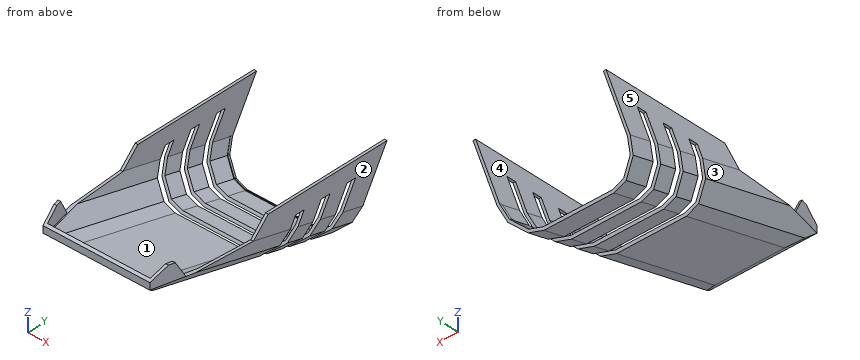
```python
from build123d import *
from OCP.BRepFilletAPI import BRepFilletAPI_MakeChamfer

# Parameters (mm, degrees)
BOSS_EXTRU_1_DEPTH                  = 500
CHANFREIN2_SIZE                     = 80
CHANFREIN3_SIZE                     = 19.999999999999996
CHANFREIN3_SIZE2                    = 38.63703305156302
CHANFREIN3_SIZE2_2                  = 38.63703305156301
CHANFREIN4_SIZE                     = 190.00000000000003
CHANFREIN4_SIZE2                    = 127.87558157978762
BOSS_EXTRU_2_DEPTH                  = 60
BOSS_EXTRU_3_DEPTH                  = 500
COQUE1_T                            = 10
ENL_V_MAT_EXTRU_2_REACH             = 940.137
ENL_V_MAT_EXTRU_2_DIRECTION_2_DEPTH = 939.1366191668232
ENL_V_START                         = -60
ENL_V_MAT_EXTRU_3_DEPTH             = 60
ENL_V_MAT_EXTRU_4_DEPTH             = 1170.3404261816813
CHANFREIN6_SIZE                     = 34.641016151
CHANFREIN6_SIZE_2                   = 60
CHANFREIN7_SIZE                     = 60
ENL_V_MAT_EXTRU_5_DEPTH             = 1170.3404261816813


# Some blends are built 0.0001 mm under size
with BuildPart() as part:
    # Esquisse3 → Boss.-Extru.1 (new body)
    with BuildSketch(Plane(origin=(0, 0, 0), x_dir=(0, 0, -1), z_dir=(1, 0, 0))):
        Polygon((0, 0), (0, 1000), (216.50635094611002, 875.0000000000006), align=None)
    extrude(amount=BOSS_EXTRU_1_DEPTH)

    # Chanfrein2
    chanfrein2_edges = [part.edges().sort_by_distance(p)[0] for p in [
        (500, 437.5000000000003, -108.25317547305501),
        (0, 437.5000000000003, -108.25317547305501),
    ]]
    chamfer(chanfrein2_edges, length=CHANFREIN2_SIZE)

    # Chanfrein3: one chamfer whose edges measure the first distance from different faces: ONE call of the kernel's chamfer builder (chamfer() names one face for all edges)
    chanfrein3_edges_1 = [part.edges().sort_by_distance(p)[0] for p in [
        (500, 624.8499399519503, -72.19766271841472),
        (420, 437.5000000000003, -108.25317547305504),
    ]]
    chanfrein3_side_1 = [part.faces().sort_by_distance(p)[0] for p in [
        (457.3358939482921, 524.9359686158087, -91.42611546732361),
    ]]
    chanfrein3_edges_2 = [part.edges().sort_by_distance(p)[0] for p in [
        (80, 437.50000000000017, -108.25317547305501),
        (0, 624.8499399519503, -72.1976627184147),
    ]]
    chanfrein3_side_2 = [part.faces().sort_by_distance(p)[0] for p in [
        (42.664106051707925, 524.9359686158089, -91.42611546732363),
    ]]
    chanfrein3 = BRepFilletAPI_MakeChamfer(part.part.solid().wrapped)
    for e in chanfrein3_edges_1:
        chanfrein3.Add(CHANFREIN3_SIZE, CHANFREIN3_SIZE2, e.wrapped, chanfrein3_side_1[0].wrapped)  # the first distance lies on this face
    for e in chanfrein3_edges_2:
        chanfrein3.Add(CHANFREIN3_SIZE, CHANFREIN3_SIZE2_2, e.wrapped, chanfrein3_side_2[0].wrapped)  # the first distance lies on this face
    add(Compound.cast(chanfrein3.Shape()), mode=Mode.REPLACE)

    # Chanfrein4
    chanfrein4_edges = [part.edges().sort_by_distance(p)[0] for p in [
        (249.99999999999994, 0, 0),
    ]]
    chanfrein4_side = [part.faces().sort_by_distance(p)[0] for p in [
        (249.99999999999997, 437.5000000000003, -108.25317547305502),
    ]]
    chamfer(chanfrein4_edges, length=CHANFREIN4_SIZE, length2=CHANFREIN4_SIZE2, reference=chanfrein4_side[0])

    # Esquisse4 → Boss.-Extru.2 (add)
    with BuildSketch(Plane.XY):
        Polygon((500, 1000), (0, 1000), (6.94e-15, 493.9253559619593), (14.142135623731011, 274.1881541390633), (49.28527880731526, 127.87558157978796), (450.7147211926849, 127.87558157978796), (485.85786437626905, 274.18815413906196), (500, 493.92535596195466), align=None)
    extrude(amount=BOSS_EXTRU_2_DEPTH)

    # Esquisse5 → Boss.-Extru.3 (add)
    with BuildSketch(Plane.ZY):
        Polygon((60, 1000), (60, 1034.6410161513777), (0, 1000), align=None)
    extrude(amount=-BOSS_EXTRU_3_DEPTH)

    # Coque1 (no face opened: a closed hollow body)
    add(offset(amount=-COQUE1_T, mode=Mode.PRIVATE), mode=Mode.SUBTRACT)

    # Esquisse6 → Enlèv. mat.-Extru.2 (cut, up to next)
    with BuildSketch(Plane(origin=(0, 750.0000000000025, -433.0127018922181), x_dir=(1, 0, 0), z_dir=(0, 0.86602540378444, -0.49999999999999784)), mode=Mode.PRIVATE) as enl_v_mat_extru_2_sk1:
        Polygon((10, -569.2820323027529), (10, -757.501187283232), (489.99999999999983, -757.5011872832318), (489.99999999999994, -569.2820323027527), (489.9999999999996, -374.7478772728107), (476.8280711810083, -323.58228852611177), (428.823967356419, -273.61803314286686), (379.9946243192759, -259.99999999999744), (120.00537568072383, -259.99999999999756), (71.17603264358065, -273.618033142867), (23.171928818991503, -323.58228852611194), (10.000000000000268, -374.74787727281085), align=None)
    enl_v_mat_extru_2_tool1 = extrude(enl_v_mat_extru_2_sk1.sketch, amount=-ENL_V_MAT_EXTRU_2_REACH, mode=Mode.PRIVATE) & part.part
    add(enl_v_mat_extru_2_tool1.solids().sort_by_distance((250, 1007.562635, 13.098868))[0], mode=Mode.SUBTRACT)

    # Esquisse6 → Enlèv. mat.-Extru.2 direction 2 (cut)
    with BuildSketch(Plane(origin=(0, 750.0000000000025, -433.0127018922181), x_dir=(1, 0, 0), z_dir=(0, 0.86602540378444, -0.49999999999999784))):
        Polygon((10, -569.2820323027529), (10, -757.501187283232), (489.99999999999983, -757.5011872832318), (489.99999999999994, -569.2820323027527), (489.9999999999996, -374.7478772728107), (476.8280711810083, -323.58228852611177), (428.823967356419, -273.61803314286686), (379.9946243192759, -259.99999999999744), (120.00537568072383, -259.99999999999756), (71.17603264358065, -273.618033142867), (23.171928818991503, -323.58228852611194), (10.000000000000268, -374.74787727281085), align=None)
    extrude(amount=ENL_V_MAT_EXTRU_2_DIRECTION_2_DEPTH, mode=Mode.SUBTRACT)

    # Esquisse7 → Enlèv. mat.-Extru.3 (cut)
    with BuildSketch(Plane.XY.offset(60).offset(ENL_V_START)):
        Polygon((475.93370620438793, 275.68803078848794), (442.8322266096682, 137.87558157978802), (57.16777339033198, 137.87558157978796), (24.066293795611983, 275.6880307884899), (10.000000000000009, 494.2468199914388), (10, 1034.6410161513777), (489.99999999999864, 1034.6410161513782), (489.9999999999996, 494.2468199914393), align=None)
    extrude(amount=ENL_V_MAT_EXTRU_3_DEPTH, mode=Mode.SUBTRACT)

    # Esquisse8 → Enlèv. mat.-Extru.4 (cut, through all)
    with BuildSketch(Plane(origin=(500, 0, 0), x_dir=(0, 0, -1), z_dir=(1, 0, 0))):
        Polygon((-60, 493.92535596195466), (0, 493.92535596195466), (-1.388e-14, 274.18815413906196), (-1.388e-14, 244.18815413906194), (-59.99999999999999, 244.18815413906194), (-60, 274.18815413906196), align=None)
    extrude(amount=-ENL_V_MAT_EXTRU_4_DEPTH, mode=Mode.SUBTRACT)

    # Chanfrein6
    # the kernel refuses this chamfer: 60, 34.641016151 mm, written as the material it takes off along each edge
    with BuildSketch(Plane(origin=(186.85746471381282, 244.1881541390619, 60), x_dir=(0, -0.9983227437537926, 0.05789386240267061), z_dir=(-1, 0, 0))) as chanfrein6_piece_1_section:
        Polygon((CHANFREIN6_SIZE * 0.998322743765, -CHANFREIN6_SIZE * 0.0578938624033), (-CHANFREIN6_SIZE_2 * 0.0578938624027, -CHANFREIN6_SIZE_2 * 0.998322743754), (0, 0), align=None)
    chanfrein6_piece_1 = extrude(amount=320.73470744761204, mode=Mode.PRIVATE)
    chanfrein6_piece_1 = split(chanfrein6_piece_1, bisect_by=Plane(origin=(26.49011099000677, 233.04123739645672, 1.648e-14), z_dir=(0, 6e-17, 1)), keep=Keep.TOP, mode=Mode.PRIVATE)
    add(chanfrein6_piece_1, mode=Mode.SUBTRACT)
    with BuildSketch(Plane(origin=(-105.93986647144428, 127.87558157978796, 60), x_dir=(0, -0.05789386240267084, -0.9983227437537926), z_dir=(1, 0, 0))) as chanfrein6_piece_2:
        Polygon((CHANFREIN6_SIZE * 0.998322743765, CHANFREIN6_SIZE * 0.0578938624033), (-CHANFREIN6_SIZE_2 * 0.0578938624027, CHANFREIN6_SIZE_2 * 0.998322743754), (0, 0), align=None)
    extrude(amount=711.8797329428887, mode=Mode.SUBTRACT)
    with BuildSketch(Plane(origin=(633.8772427337997, 244.1881541390619, 60), x_dir=(0, -0.9983227437537926, 0.05789386240267061), z_dir=(-1, 0, 0))) as chanfrein6_piece_3_section:
        Polygon((CHANFREIN6_SIZE * 0.998322743765, -CHANFREIN6_SIZE * 0.0578938624033), (-CHANFREIN6_SIZE_2 * 0.0578938624027, -CHANFREIN6_SIZE_2 * 0.998322743754), (0, 0), align=None)
    chanfrein6_piece_3 = extrude(amount=320.7347074476121, mode=Mode.PRIVATE)
    chanfrein6_piece_3 = split(chanfrein6_piece_3, bisect_by=Plane(origin=(473.5098890099937, 233.04123739645678, 1.648e-14), z_dir=(0, 6e-17, 1)), keep=Keep.TOP, mode=Mode.PRIVATE)
    add(chanfrein6_piece_3, mode=Mode.SUBTRACT)

    # Chanfrein7
    chanfrein7_edges = [part.edges().sort_by_distance(p)[0] for p in [
        (5.010344602246278, 493.92535596195466, 60),
        (494.98965539775355, 493.92535596195466, 60),
    ]]
    chamfer(chanfrein7_edges, length=CHANFREIN7_SIZE - 0.0001)  # a hair under: the kernel refuses the full size

    # Esquisse10 → Enlèv. mat.-Extru.5 (cut, through all)
    with BuildSketch(Plane(origin=(500, 0, 0), x_dir=(0, 0, -1), z_dir=(1, 0, 0))):
        Polygon((196.50635094610988, 794.1709623134528), (2.06e-15, 907.6239569296604), (4.01e-15, 872.9829407782828), (189.0063509461099, 763.8600731809975), align=None)
        Polygon((174.00635094610982, 703.2382949160867), (1.402e-14, 803.7009084755275), (1.911e-14, 769.0598923241499), (166.50635094610982, 672.9274057836313), align=None)
        Polygon((151.50635094610985, 612.3056275187206), (2.603e-14, 699.7778600213949), (3.259e-14, 665.1368438700174), (144.00635094610985, 581.9947383862652), align=None)
    extrude(amount=-ENL_V_MAT_EXTRU_5_DEPTH, mode=Mode.SUBTRACT)


solid = part.part
```
Geometry: final body of the model. Coordinates: model frame, mm. Face numbers are marked on the shaded views. A direction names the side the tool comes from. Coordinates: 2 decimals unless noted, no trailing zeros. Order: outer loops, then holes, each group sorted by start corner. A loop starts at its lowest first (then second) coordinate and runs counter-clockwise, first axis right, second up. Notation, with made-up numbers: (55, 45.5) -> (89, 45.5) arc R21 cw to (89, 73.5) -> close; hole circle Ø11 at (54, -4). An arc over 180 degrees is marked (long way). Write item = value, one per line.
(1) Pin query (flat end, axial travel): pin 1 Ø25 at (x, z) = (278.5, 11.5) entering from +Y; pin 2 Ø4 at (x, z) = (408.5, -127.5) entering from +Y; pin 3 Ø1 at (y, z) = (865.5, -109.5) entering from +X. Return the tip coordinate at first contact, or that it passes through.
Solved:
pin_1 = 145.04
pin_2 = 591.44
pin_3 = 495.57
(2) Cut plane D-D on y = 306. Return loops of the section in (x, z), plus the area to 3 significant figures.
Solved:
outline = (12.09, 0) -> (14.14, -7.87) -> (65.86, -61.15) -> (118.64, -75.72) -> (381.36, -75.72) -> (434.14, -61.15) -> (485.86, -7.87) -> (487.91, 0) -> (477.55, 0) -> (476.89, -2.54) -> (428.97, -51.91) -> (380.05, -65.41) -> (119.95, -65.41) -> (71.03, -51.91) -> (23.11, -2.54) -> (22.45, 0) -> close
area = 5,340 mm²
(3) Line query: line 1 (X direction, y = 849, z = 2); line 2 (Y direction, x = 249, z = 17.5); line 3 (X direction, y = 478.5, z = -43.5). Output: solid intervals per line, ascending.
Solved:
line_1 = 0 to 10, 490 to 500
line_2 = 127.88 to 137.88
line_3 = 12.31 to 22.66, 477.34 to 487.69
(4) Cut plane B-B on z = 13. Return loops of the section in (x, y), plus the area to 3 significant figures.
Solved:
outline = (0, 506.93) -> (10, 506.93) -> (10, 1007.51) -> (0, 1007.51) -> close; (23.15, 236.68) -> (49.29, 127.88) -> (450.71, 127.88) -> (476.85, 236.68) -> (466.56, 236.68) -> (442.83, 137.88) -> (57.17, 137.88) -> (33.44, 236.68) -> close; (490, 506.93) -> (500, 506.93) -> (500, 1007.51) -> (490, 1007.51) -> close
area = 16,100 mm²
(5) Cut plane C-C on y = 842.5. Return loops of the section in (x, z).
Solved:
outline = (0, -52.8) -> (10, -52.8) -> (10, 60) -> (0, 60) -> close; (6.91, -112.8) -> (14.14, -140.62) -> (65.86, -193.9) -> (118.64, -208.46) -> (381.36, -208.46) -> (434.14, -193.9) -> (485.86, -140.62) -> (493.09, -112.8) -> (482.74, -112.8) -> (476.89, -135.29) -> (428.97, -184.66) -> (380.05, -198.16) -> (119.95, -198.16) -> (71.03, -184.66) -> (23.11, -135.29) -> (17.26, -112.8) -> close; (490, -52.8) -> (500, -52.8) -> (500, 60) -> (490, 60) -> close
(6) Cut plane A-A on x = 220. Return loops of the section in (y, z).
Solved:
outline = (127.88, 0) -> (184.44, -45.64) -> (581.99, -144.01) -> (587.2, -134.99) -> (188.99, -36.46) -> (143.8, 0) -> (137.88, 0) -> (137.88, 31.13) -> (127.88, 25.36) -> close; (612.31, -151.51) -> (672.93, -166.51) -> (678.13, -157.49) -> (617.51, -142.49) -> close; (703.24, -174.01) -> (763.86, -189.01) -> (769.06, -179.99) -> (708.44, -164.99) -> close; (794.17, -196.51) -> (875, -216.51) -> (880, -207.85) -> (871.34, -202.85) -> (870.1, -204.99) -> (799.38, -187.49) -> close
(7) Access query for the marked faces 4 and 5. Directions: +Z, -Z, +X, -X, +Y, -Y. A direction counts if a zero-diameter tool reaches every point of the face in a straight line with its end or side. Return the directions, or none.
Solved:
face_4 = +Z, +Y
face_5 = +Z, -Z, -X, +Y, -Y
(8) Pull-direction query (X, two-part tool) for the marked faces 1, 2 and 3; classes: pulls with the +X half, pulls with the -X half, needs draft (parallel to the pull), parting line crosses it, or undercut.
Solved:
face_1 = undercut
face_2 = pulls with the +X half
face_3 = pulls with the -X half
